Check sheet for the modelled part. Datum: model origin and axes. Units: mm. Face numbers are marked on the shaded views. A direction names the side the tool comes from. Coordinates: 2 decimals unless noted, no trailing zeros. Order: outer loops, then holes, each group sorted by start corner. A loop starts at its lowest first (then second) coordinate and runs counter-clockwise, first axis right, second up.
from build123d import *

# Parameters (mm, degrees)
SKETCH_1_R      = 4
EXTRUDE_1_DEPTH = 20
SKETCH_2_R      = 3.15
SKETCH_4_R      = 8
EXTRUDE_2_DEPTH = 5


with BuildPart() as part:
    # ｽｹｯﾁ1 → ﾎﾞｽ - 押し出し1 (new body)
    with BuildSketch(Plane.XY):
        Circle(SKETCH_1_R)
    extrude(amount=EXTRUDE_1_DEPTH)

    # ｽｲｰﾌﾟ1: sweep along a path in ｽｹｯﾁ3
    with BuildLine(Plane(origin=(0, 0, 0), x_dir=(0, 0, -1), z_dir=(1, 0, 0))) as sweep_1_path:
        CenterArc((-33.15, 0), 13.15, 0, 360)
    # ｽｹｯﾁ2 → ｽｲｰﾌﾟ1 (sweep)
    with BuildSketch(Plane(origin=(0, 0, 0), x_dir=(1, 0, 0), z_dir=(0, 1, 0))):
        with Locations((0, -20)):
            Circle(SKETCH_2_R)
    sweep(path=sweep_1_path.line)

    # ｽｹｯﾁ4 → ﾎﾞｽ - 押し出し2 (add, symmetric)
    with BuildSketch(Plane(origin=(0, 0, 15), x_dir=(-1, 0, 0), z_dir=(0, 0, -1))):
        Circle(SKETCH_4_R)
    extrude(amount=EXTRUDE_2_DEPTH, both=True)


solid = part.part
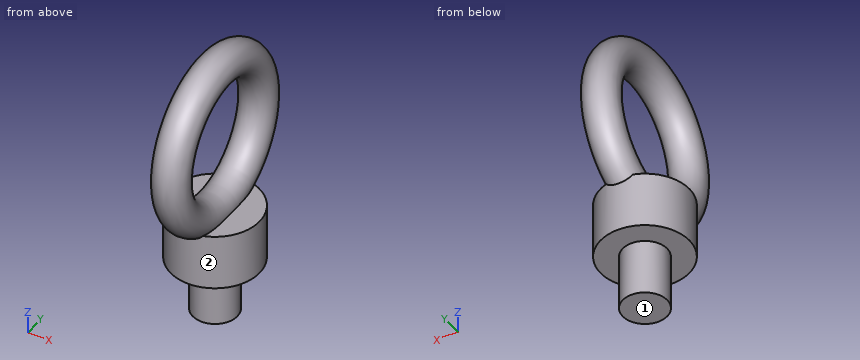
(1) Cross-section at C-C (x = 5.75). Enter the section's corners in (y, z).
Filled in:
outline: (-5.56, 10) - (5.56, 10) - (5.56, 20) - (-5.56, 20) - close
(2) Tool access check on the marked faces 1 and 2. Record the directions out of +Z, -Z, +X, -X, +Y, -Y that give a thin tool (end or side, any length) a straight path to the whole face; none if there is none.
Filled in:
face 1: -Z, +X, -X, +Y, -Y
face 2: -Z
(3) Cross-section at A-A (x = 0). Enter the section's corners in (y, z), and give its area (3 significant figures).
Filled in:
outline: (-8, 10) - (-4, 10) - (-4, 0) - (4, 0) - (4, 10) - (8, 10) - (8, 18.95) arc R16.3 ccw (long way) to (-8, 18.95) - close; hole circle Ø20 at (0, 33.15)
area: 721 mm2
(4) Thickness scan on probe 1 along Z at (x, y) = (1, 5); probe 2 along Z at (x, y) = (1, 3); probe 3 along Z at (x, y) = (-3.25, -4). Record the ranges inside material, lowest first.
Filled in:
probe 1: z = 10 to 24.3, 42 to 48.49
probe 2: z = 0 to 23.44, 42.86 to 49.01
probe 3: z = 10 to 20
(5) Cross-section at D-D (x = -6.5). Enter the section's corners in (y, z), and give its area (3 significant figures).
Filled in:
outline: (-4.66, 10) - (4.66, 10) - (4.66, 20) - (-4.66, 20) - close
area: 93.3 mm2
(6) Go/stop test with flat-tipped pins: P1, Ø5, axis at y = 1.5, z = 42, coming from the -X side; P2, Ø10, axis at y = -11, z = 11, coming from the +X side; P3, Ø6, axis at x = 5.5, z = 41.5, coming from the +Y side. Record where each tip stops, or that it passes through.
Filled in:
P1: stops at x = -2.67
P2: stops at x = 5.29
P3: stops at y = 12.87
(7) Cross-section at B-B (z = 3). Enter the section's corners in (x, y), and give its area (3 significant figures).
Filled in:
outline: circle Ø8 at (0, 0)
area: 50.3 mm2
